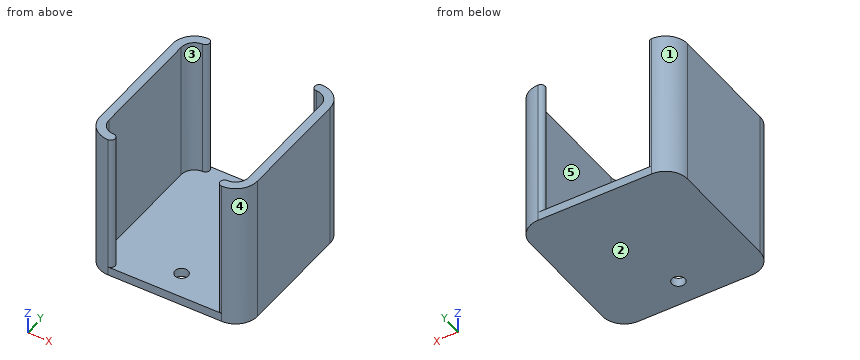
from build123d import *

# Parameters (mm, degrees)
F0_W     = 36
F0_H     = 36
F1_DEPTH = 34
F2_R     = 5
F4_DEPTH = 32
F5_R     = 1.5
F6_DEPTH = 25
F8_DEPTH = 32


with BuildPart() as f1:
    # F0 (on Top) → F1 (new body)
    with BuildSketch(Plane.XY):
        Rectangle(F0_W, F0_H)
    extrude(amount=F1_DEPTH)

    # F2
    f2_edges = [f1.edges().sort_by_distance(p)[0] for p in [
        (18, 18, 17),
        (-18, 18, 17),
        (18, -18, 17),
        (-18, -18, 17),
    ]]
    fillet(f2_edges, radius=F2_R)

    # F3 (on face) → F4 (cut)
    with BuildSketch(Plane.XY.offset(34)):
        with BuildLine():
            ThreePointArc((-13, 18), (-12, 17), (-13, 16))
            ThreePointArc((-13, 16), (-15.1213203436, 15.1213203436), (-16, 13))
            Line((-16, 13), (-16, -13))
            ThreePointArc((-16, -13), (-15.1213203436, -15.1213203436), (-13, -16))
            Line((-13, -16), (13, -16))
            ThreePointArc((13, -16), (15.1213203436, -15.1213203436), (16, -13))
            Line((16, -13), (16, 13))
            ThreePointArc((16, 13), (15.1213203436, 15.1213203436), (13, 16))
            ThreePointArc((13, 16), (12, 17), (13, 18))
            Line((13, 18), (-13, 18))
        make_face()
    extrude(amount=-F4_DEPTH, mode=Mode.SUBTRACT)

    # F5 (on face) → F6 (cut)
    with BuildSketch(Plane(origin=(0, 0, 0), x_dir=(1, 0, 0), z_dir=(0, 0, -1))):
        with Locations((0, 12)):
            Circle(F5_R)
    extrude(amount=-F6_DEPTH, mode=Mode.SUBTRACT)

    # F7 (on face) → F8 (cut, through all)
    with BuildSketch(Plane.XY.offset(34)):
        with BuildLine():
            ThreePointArc((-13, -16), (-12, -17), (-13, -18))
            Line((-13, -18), (13, -18))
            ThreePointArc((13, -18), (12, -17), (13, -16))
            Line((13, -16), (-13, -16))
        make_face()
    extrude(amount=-F8_DEPTH, mode=Mode.SUBTRACT)


solid = f1.part
The model under review builds one solid part; all positions refer to its coordinate system, in mm. Face numbers are marked on the shaded views. A direction names the side the tool comes from. Give positions to 0.01 mm unless a question says otherwise; leave off trailing zeros. Write each loop counter-clockwise with the first axis right and the second up, starting at its lowest first coordinate (ties: lowest second). Pieces come first, ordered by that corner, then holes.
1. Add section B-B, the plane z = 17.5. Write out the cut boundary in (x, y).
2. Add section C-C, the plane y = 7.5. Write out the cut boundary in (x, z).
3. Add section A-A, the plane y = -12. Write out the cut boundary in (x, z).
4. Add section D-D, the plane y = 17. Write out the cut boundary in (x, z), plus the area to 3 significant figures.
5. For P1, Ø8, axis at x = -0.5, y = -4.5, coming from the -Z side; P2, Ø9.5, axis at x = -3, y = -8, coming from the +Z side, all flat-tipped, find the tip position at first contact; note any pin that passes through.
6. Tool access review of the marked faces 4 and 5: name each direction out of +Z, -Z, +X, -X, +Y, -Y from which nothing blocks a thin tool from reaching the whole face with its end or side.
7. Draft analysis for pull direction X (two halves, no side actions). For the marked faces 1, 2 and 3, state which applies: +X half, -X half, draft (parallel to the pull), parting line (faces both ways), or undercut.
8. Wall thickness on L1, parallel to X at y = -6, z = 30; L2, parallel to X at y = -12, z = 1.35; L3, parallel to Y at x = 0, z = 0.65: over which ranges is each line inside the solid? List them lowest first.
Worked answers:
1. outline: (-18, -13) arc R5 ccw to (-13, -18) arc R1 ccw to (-13, -16) arc R3 cw to (-16, -13) - (-16, 13) arc R3 cw to (-13, 16) arc R1 ccw to (-13, 18) arc R5 ccw to (-18, 13) - close; (13, -18) arc R5 ccw to (18, -13) - (18, 13) arc R5 ccw to (13, 18) arc R1 ccw to (13, 16) arc R3 cw to (16, 13) - (16, -13) arc R3 cw to (13, -16) arc R1 ccw to start
2. outline: (-18, 0) - (18, 0) - (18, 34) - (16, 34) - (16, 2) - (-16, 2) - (-16, 34) - (-18, 34) - close
3. outline: (-18, 0) - (-1.5, 0) - (-1.5, 2) - (-16, 2) - (-16, 34) - (-18, 34) - close; (1.5, 0) - (18, 0) - (18, 34) - (16, 34) - (16, 2) - (1.5, 2) - close
4. outline: (-16, 0) - (16, 0) - (16, 34) - (12, 34) - (12, 2) - (-12, 2) - (-12, 34) - (-16, 34) - close
4. area: 320 mm2
5. P1: stops at z = 0
5. P2: stops at z = 2
6. face 4: +Z, -Z, +X, -Y
6. face 5: +Z
7. face 1: -X half
7. face 2: draft
7. face 3: undercut
8. L1: x = -18 to -16, 16 to 18
8. L2: x = -18 to -1.5, 1.5 to 18
8. L3: y = -18 to -13.5, -10.5 to 18
